For this review, use the dimensioned drawing (mm, ordinates from the lowest corner) and the shaded views. A direction names the side the tool comes from. Give positions to 0.01 mm unless a question says otherwise; leave off trailing zeros. Loops run counter-clockwise (first coordinate to the right, second up) from the corner with the lowest first, then second, coordinate; pieces in that order, holes last. Notation, with made-up numbers: M 89.25,34.5 L 143.25,34.5 A26 cw 143.25,55.5 Z; hole C 73,-34.5 d10. An arc over 180 degrees is marked long. Use CSV: the item, a comma, the result in double quotes.
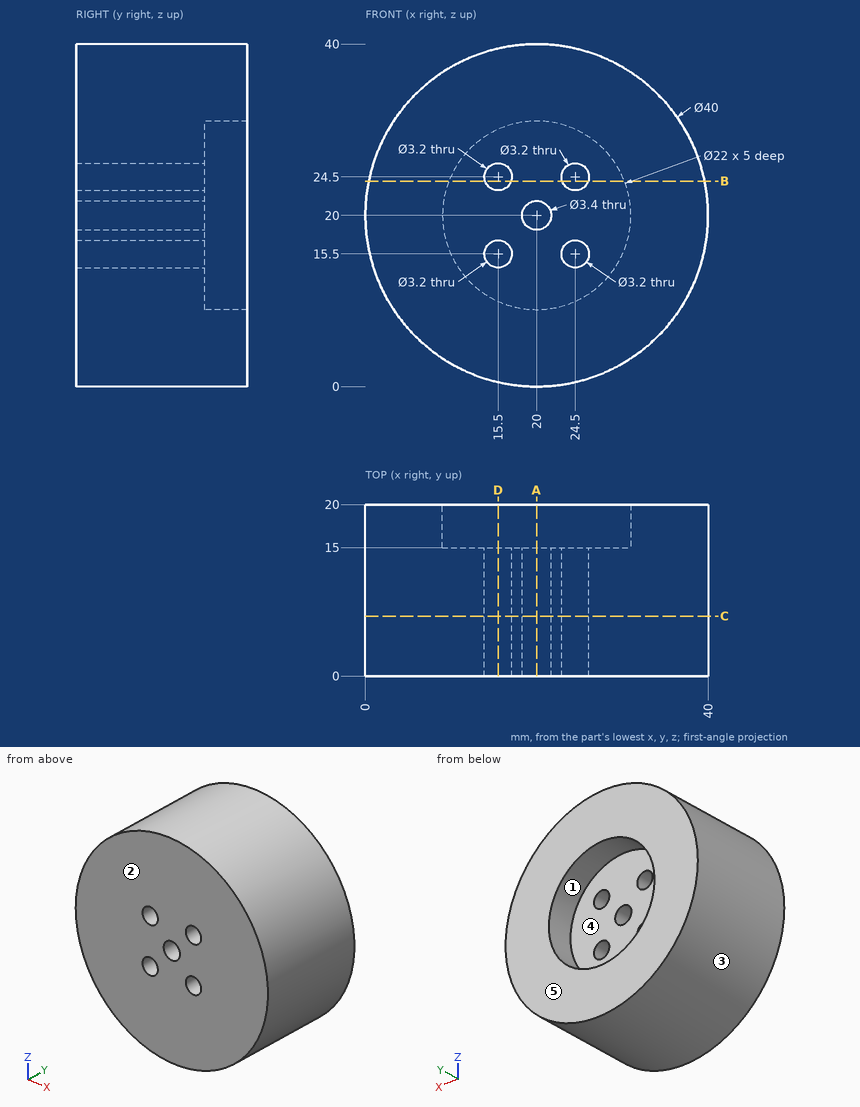
(1) Wall thickness on line 1 along Z through (x, y) = (24.5, 9.5); line 2 along X through (y, z) = (9.75, 24); line 3 along Z through (x, y) = (20, 18.05): over which ranges is each line inside the solid? List them lowest first. Write a range as [from, to].
A:
line 1,"[0.51, 13.9], [17.1, 22.9], [26.1, 39.49]"
line 2,"[0.4, 13.98], [17.02, 22.98], [26.02, 39.6]"
line 3,"[0, 9], [31, 40]"
(2) We need section A-A on x = 20. State the section outline as (y, z) points.
A:
outline,"M 0,0 L 20,0 L 20,9 L 15,9 L 15,18.3 L 0,18.3 Z; M 0,21.7 L 15,21.7 L 15,31 L 20,31 L 20,40 L 0,40 Z"
(3) Clearance check with flat-ended pins moving along their axes: P1, Ø5.5, axis at x = 20, z = 20, coming from the +Y side; P2, Ø2.5, axis at x = 15.5, z = 24.5, coming from the -Y side; P3, Ø5, axis at x = 30.5, y = 15, coming from the -Z side; P4, Ø8, axis at x = 8.5, y = 7.5, coming from the +Z side. State where each tip first meets the part, or that it passes through.
A:
P1,"y = 15"
P2,"through"
P3,"z = 1.67"
P4,"z = 38.54"
(4) The part is to be moulded in two halves that separate along Z. For the marked faces 3, 4 and 5, say which applies: released by +Z, released by -Z, zero draft, split by the parting line, or undercut.
A:
face 3,"split by the parting line"
face 4,"undercut"
face 5,"zero draft"
(5) We need section D-D on x = 15.5. State the section outline as (y, z) points.
A:
outline,"M 0,0.51 L 20,0.51 L 20,9.96 L 15,9.96 L 15,13.9 L 0,13.9 Z; M 0,17.1 L 15,17.1 L 15,22.9 L 0,22.9 Z; M 0,26.1 L 15,26.1 L 15,30.04 L 20,30.04 L 20,39.49 L 0,39.49 Z"
(6) We need section C-C on y = 7. State the section outline as (x, z) points.
A:
outline,"C 20,20 d40; hole C 15.5,15.5 d3.2; hole C 15.5,24.5 d3.2; hole C 20,20 d3.4; hole C 24.5,15.5 d3.2; hole C 24.5,24.5 d3.2"
(7) We need section B-B on z = 24. State the section outline as (x, y) points, then the cut area to 3 significant figures.
A:
outline,"M 0.4,0 L 13.98,0 L 13.98,15 L 9.75,15 L 9.75,20 L 0.4,20 Z; M 17.02,0 L 22.98,0 L 22.98,15 L 17.02,15 Z; M 26.02,0 L 39.6,0 L 39.6,20 L 30.25,20 L 30.25,15 L 26.02,15 Z"
area,"590 mm²"
(8) Machinability: for the marked faces 1 and 2, which of the approach directions +Z, -Z, +X, -X, +Y, -Y give a long, thin tool a straight path to every point of the face, cutting with its end or side? Answer none if there is none.
A:
face 1,"+Y"
face 2,"+Z, -Z, +X, -X, -Y"
